Source: CAD feature listing. Evaluate the final solid. Frame: model axes, mm. Face numbers are marked on the shaded views. A direction names the side the tool comes from. Give positions to 0.01 mm unless a question says otherwise; leave off trailing zeros. Order: outer loops, then holes, each group sorted by start corner. A loop starts at its lowest first (then second) coordinate and runs counter-clockwise, first axis right, second up.
```python
from build123d import *

# Parameters (mm, degrees)
F1_W     = 15
F1_H     = 27.4107800126
F1_R     = 4.25
F1_H_2   = 3.5892199874
F1_H_3   = 4
F2_DEPTH = 17
F3_DEPTH = 2
F4_START = -15
F1_H_4   = 4.0437440276
F4_DEPTH = 2
F5_R     = 3
F0_R     = 1.55
F6_DEPTH = 25
F7_START = 2
F0_R_2   = 3.8628325464
F7_DEPTH = 23
F8_SIZE  = 2
F9_R     = 0.5


with BuildPart() as f2:
    # F1 (on Right) → F2 (new body)
    with BuildSketch(Plane.YZ):
        Polygon((-1.5120996646, 0), (0, 0), (0, 28), (-15, 28), (-15, 55.4107800126), (-33.6045285314, 55.4107800126), align=None)
        with Locations((-7.5, 41.7053900063)):
            Rectangle(F1_W, F1_H)
        with Locations((-8, 44)):
            Circle(F1_R, mode=Mode.SUBTRACT)
        with Locations((-7.5, 57.2053900063)):
            Rectangle(F1_W, F1_H_2)
        Polygon((-35.6833079152, 59), (-33.6045285314, 55.4107800126), (-15, 55.4107800126), (-15, 59), align=None)
        Polygon((-38, 63), (-35.6833079152, 59), (-15, 59), (-15, 63), align=None)
        with Locations((-7.5, 61)):
            Rectangle(F1_W, F1_H_3)
        Polygon((-156.0687124729, 59), (-35.6833079152, 59), (-38, 63), (-190, 63), (-190, 59), align=None)
        Polygon((-169.6997248952, 35.7001498342), (-156.0687124729, 59), (-190, 59), (-190, 35.7001498342), align=None)
        Polygon((-173.0344593525, 30), (-169.6997248952, 35.7001498342), (-190, 35.7001498342), (-190, 30), align=None)
    extrude(amount=-F2_DEPTH)

    # F1 (on Right) → F3 (cut)
    with BuildSketch(Plane.YZ):
        with Locations((-7.5, 41.7053900063)):
            Rectangle(F1_W, F1_H)
        with Locations((-8, 44)):
            Circle(F1_R, mode=Mode.SUBTRACT)
        with Locations((-7.5, 57.2053900063)):
            Rectangle(F1_W, F1_H_2)
        with Locations((-7.5, 61)):
            Rectangle(F1_W, F1_H_3)
    extrude(amount=-F3_DEPTH, mode=Mode.SUBTRACT)

    # F1 (on Right) → F4 (join)
    with BuildSketch(Plane.YZ.offset(F4_START)):
        Polygon((-190, 63), (-38, 63), (-15, 63), (-15, 67.0437440276), (-190, 67.0437440276), align=None)
        with Locations((-7.5, 65.0218720138)):
            Rectangle(F1_W, F1_H_4)
    extrude(amount=-F4_DEPTH)

    # F5
    f5_edges = [f2.edges().sort_by_distance(p)[0] for p in [
        (-1, -15, 28),
        (-1, -15, 63),
        (-1, 0, 28),
    ]]
    fillet(f5_edges, radius=F5_R)

    # F0 (on Front) → F6 (cut)
    with BuildSketch(Plane.XZ):
        with Locations((-7, 8)):
            Circle(F0_R)
    extrude(amount=F6_DEPTH, mode=Mode.SUBTRACT)

    # F0 (on Front) → F7 (cut)
    with BuildSketch(Plane.XZ.offset(F7_START)):
        with Locations((-7, 8)):
            Circle(F0_R_2)
        with Locations((-7, 8)):
            Circle(F0_R, mode=Mode.SUBTRACT)
    extrude(amount=F7_DEPTH, mode=Mode.SUBTRACT)

    # F8
    f8_edges = [f2.edges().sort_by_distance(p)[0] for p in [
        (-17, -18.597704, 29.5),
        (-17, -95.87601, 59),
        (-17, -164.551586, 44.5),
        (-17, -190, 48.521872),
    ]]
    chamfer(f8_edges, length=F8_SIZE)

    # F9
    f9_edges = [f2.edges().sort_by_distance(p)[0] for p in [
        (-15, -95, 63),
        (-15, -95, 67.043744),
        (-17, -94, 67.043744),
        (-16, -189, 67.043744),
        (-16, 0, 67.043744),
        (-17, -12.25, 44),
    ]]
    fillet(f9_edges, radius=F9_R)


solid = f2.part
```
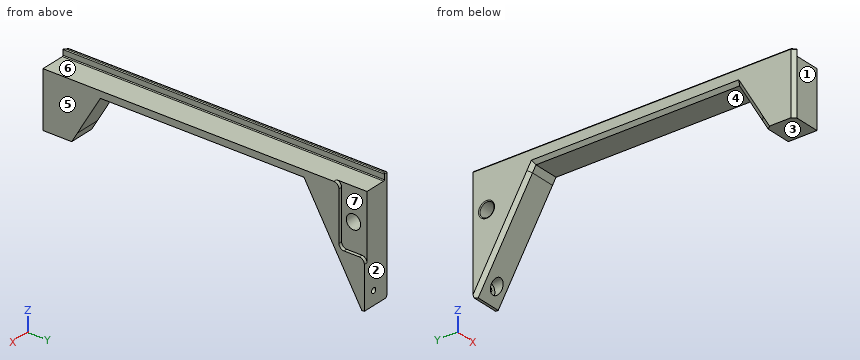
1) Material intervals for L1, parallel to X at y = -3, z = 8; L2, parallel to Z at x = -7, y = -0.6; L3, parallel to Z at x = -5, y = -176.5, sorted ascending.
Report:
L1: x = -17 to -10.86, -3.14 to 0
L2: z = 0 to 6.45, 9.55 to 63
L3: z = 30 to 63
2) Section query A-A, the plane z = 44. Return the cut outline in (x, y).
Report:
outline: (-17, -188) - (-15, -190) - (0, -190) - (0, -164.84) - (-15, -164.84) - (-17, -167.16) - close; (-17, -24.68) - (-15, -27) - (0, -27) - (0, -15) - (-2, -15) - (-2, -12.25) - (-16.5, -12.25) arc R0.5 ccw to (-17, -12.75) - close; (-17, -3.25) arc R0.5 ccw to (-16.5, -3.75) - (-2, -3.75) - (-2, 0) - (-17, 0) - close
3) Section query C-C, the plane y = -162.5. Return the cut outline in (x, z).
Report:
outline: (-17, 51.97) - (-15, 48.01) - (0, 48.01) - (0, 63) - (-14.5, 63) arc R0.5 cw to (-15, 63.5) - (-15, 66.54) arc R0.5 ccw to (-15.5, 67.04) - (-16.5, 67.04) arc R0.5 ccw to (-17, 66.54) - close
4) Pin query (flat end, axial travel): pin 1 (0.6 mm diameter, centred on x = -1, z = 38.5, fed in from +Y); pin 2 (2.5 mm diameter, centred on x = -7, z = 8, fed in from +Y); pin 3 (4.5 mm diameter, centred on x = -6.5, y = -68, fed in from -Z); pin 4 (0.9 mm diameter, centred on y = -61, z = 65.5, fed in from +X). Return the tip coordinate at first contact, or that it passes through.
Report:
pin 1: stops at y = -15
pin 2: passes through
pin 3: stops at z = 59
pin 4: stops at x = -15
5) Section query B-B, the plane y = -92. Return the cut outline in (x, z), and give its area (3 significant figures).
Report:
outline: (-17, 61) - (-15, 59) - (0, 59) - (0, 63) - (-14.5, 63) arc R0.5 cw to (-15, 63.5) - (-15, 66.54) arc R0.5 ccw to (-15.5, 67.04) - (-16.5, 67.04) arc R0.5 ccw to (-17, 66.54) - close
area: 74.0 mm2
6) Section query D-D, the plane z = 15.5. Return the cut outline in (x, y), and give its area (3 significant figures).
Report:
outline: (-17, -8.18) - (-15, -10.49) - (0, -10.49) - (0, 0) - (-17, 0) - close
area: 176 mm2
7) Reachability of the marked faces 5, 6 and 7 from +Z, -Z, +X, -X, +Y, -Y: full face, straight path, thin tool, end or side. Return the list, or none.
Report:
face 5: +Z, -Z, +X, +Y, -Y
face 6: +Z, +X, +Y, -Y
face 7: +Z, +X, +Y
8) Draft query along Y for the marked faces 1, 2, 3 and 4. Return one class per face: +Y half, -Y half, draft (parallel to the pull), parting line (faces both ways), or undercut.
Report:
face 1: -Y half
face 2: +Y half
face 3: draft
face 4: undercut
